Read the model definition and answer for the solid it produces. Units are mm, in the model's axes. A direction names the side the tool comes from. Coordinates: 2 decimals unless noted, no trailing zeros. Order: outer loops, then holes, each group sorted by start corner. A loop starts at its lowest first (then second) coordinate and runs counter-clockwise, first axis right, second up. Notation, with made-up numbers: (14.5, -35) -> (25.5, -35) arc R12 ccw to (25.5, -21) -> close; hole circle Ø11 at (85.25, 54). An arc over 180 degrees is marked (long way). Return JSON: item names as keys, results as strings. Group by question number.
```python
from build123d import *

# Parameters (mm, degrees)
BOX002_W        = 88.9
BOX002_H        = 88.9
BOX002_DEPTH    = 2438.4
SKETCH_W        = 38.1
SKETCH_H        = 88.9
POCKET_DEPTH    = 88.9010000032
POCKET006_DEPTH = 88.901
POCKET012_DEPTH = 38.1
SKETCH017_W     = 38.1
SKETCH017_H     = 111.76
POCKET014_DEPTH = 88.901
SKETCH034_W     = 88.9
SKETCH034_H     = 88.9
POCKET024_DEPTH = 38.1


with BuildPart() as obj1:
    # Box002 → Box002 (new body)
    with BuildSketch(Plane(origin=(1435.1, 0, 0), x_dir=(1, 0, 0), z_dir=(0, 0, 1))):
        with Locations((44.45, 44.45)):
            Rectangle(BOX002_W, BOX002_H)
    extrude(amount=BOX002_DEPTH)

    # Sketch → Pocket (cut, through all)
    with BuildSketch(Plane(origin=(1435.1, 0, 0), x_dir=(1, 0, 0), z_dir=(0, -1, 0))):
        with Locations((69.85, 501.65)):
            Rectangle(SKETCH_W, SKETCH_H)
    extrude(amount=-POCKET_DEPTH, mode=Mode.SUBTRACT)


with BuildPart() as pocket024:
    # Part__Mirroring001: instance of obj1
    add(obj1.part.mirror(Plane(origin=(762, 0, 0), x_dir=(0, -1, 0), z_dir=(1, 0, 0))))

    # Sketch007 → Pocket006 (cut, through all)
    with BuildSketch(Plane.YZ.offset(88.9)):
        Polygon((0, 1667.24584), (0, 2438.4), (88.9, 2438.4), (88.9, 1699.6027938263), align=None)
    extrude(amount=-POCKET006_DEPTH, mode=Mode.SUBTRACT)

    # Sketch013 → Pocket012 (cut)
    with BuildSketch(Plane(origin=(0, 0, 0), x_dir=(0, -1, 0), z_dir=(-1, 0, 0))):
        Polygon((-88.9, 1699.6109218263), (-88.9, 1559.9109218263), (0, 1527.553968), (0, 1667.253968), align=None)
    extrude(amount=-POCKET012_DEPTH, mode=Mode.SUBTRACT)

    # Sketch017 → Pocket014 (cut, through all)
    with BuildSketch(Plane.YZ.offset(88.9)):
        with Locations((19.05, 1633.855)):
            Rectangle(SKETCH017_W, SKETCH017_H)
    extrude(amount=-POCKET014_DEPTH, mode=Mode.SUBTRACT)

    # Sketch034 → Pocket024 (cut)
    with BuildSketch(Plane(origin=(0, 0, 0), x_dir=(0, -1, 0), z_dir=(-1, 0, 0))):
        with Locations((-44.45, 1085.85)):
            Rectangle(SKETCH034_W, SKETCH034_H)
    extrude(amount=-POCKET024_DEPTH, mode=Mode.SUBTRACT)


solid = pocket024.part
```
1. Which of the six approach directions +Z, -Z, +X, -X, +Y, -Y give full straight-line access (tool end or side, diameter ignored) to faces 4 (the face through (19, 45, 1041.4)), 5 (the face through (64, 19, 1577.975)), 6 (the face through (0, 44, 790))?
2. Find section A-A on x = 23. Determine the outline of the cut face in (y, z), and give its area (3 significant figures).
3. Straight lines are drawn through the part: L1, parallel to Z at x = 7, y = 49; L2, parallel to Z at x = 33, y = 6; L3, parallel to Z at x = 47, y = 36 (3 decimals). For each, find the intervals that lie inside material, in ascending order.
4. For a pull along Z with two mould halves and no side action, classify faces 1 (the face through (38.1, 44, 501)), 2 (the face through (18.78, 45.07, 1543.96)), 3 (the face through (38.1, 55, 1615)) as released by +Z, released by -Z, zero draft, split by the parting line, or undercut.
5. Find section B-B on y = 65. Determine the outline of the cut face in (x, z).
6. Given pin 1 (11.5 mm diameter, centred on x = 17.5, y = 60.5, fed in from +Z); pin 2 (11.5 mm diameter, centred on x = 61.5, y = 11, fed in from +Z) (3 decimals); pin 3 (15 mm diameter, centred on x = 70.5, z = 1630.5, fed in from -Y), each flat-ended and moving along its own axis, determine where each tip first touches the part or whether it passes through.
Result:
{
 "1": {"face 4": "-X, +Y, -Y", "face 5": "+Z, +X, -X, -Y", "face 6": "+Z, -Z, -X, +Y, -Y"},
 "2": {"outline": "(0, 0) -> (88.9, 0) -> (88.9, 457.2) -> (0, 457.2) -> close; (0, 546.1) -> (88.9, 546.1) -> (88.9, 1041.4) -> (0, 1041.4) -> close; (0, 1130.3) -> (88.9, 1130.3) -> (88.9, 1559.91) -> (0, 1527.55) -> close", "area": "121,000 mm^2"},
 "3": {"L1": "0 to 457.2, 546.1 to 1041.4, 1130.3 to 1545.39", "L2": "0 to 457.2, 546.1 to 1041.4, 1130.3 to 1529.74", "L3": "0 to 1577.975"},
 "4": {"face 1": "undercut", "face 2": "released by +Z", "face 3": "zero draft"},
 "5": {"outline": "(0, 0) -> (88.9, 0) -> (88.9, 1690.9) -> (38.1, 1690.9) -> (38.1, 1551.21) -> (0, 1551.21) -> (0, 1130.3) -> (38.1, 1130.3) -> (38.1, 1041.4) -> (0, 1041.4) -> (0, 546.1) -> (38.1, 546.1) -> (38.1, 457.2) -> (0, 457.2) -> close"},
 "6": {"pin 1": "z = 1551.67", "pin 2": "z = 1577.975", "pin 3": "y = 38.1"}
}
